Geometry: final body of the model. Coordinates: model frame, mm. Face numbers are marked on the shaded views. A direction names the side the tool comes from. Give positions to 0.01 mm unless a question says otherwise; leave off trailing zeros. Order: outer loops, then holes, each group sorted by start corner. A loop starts at its lowest first (then second) coordinate and runs counter-clockwise, first axis right, second up. Notation, with made-up numbers: (4.25, -16) - (42.25, -16) arc R11 ccw to (42.25, -1) - close; hole circle Ø6 at (33.25, 57). An arc over 180 degrees is marked (long way). One line per item, written item: value.
```python
from build123d import *

# Parameters (mm, degrees)
SKETCH1_R                       = 15.5
BASE_FLANGE1_DEPTH              = 2
EDGE_FLANGE1_STRIP_W            = 9.4732
EDGE_FLANGE1_STRIP_H            = 2
EDGE_FLANGE1_STRIP_CUT_DEPTH    = 40
EDGE_FLANGE1_RELIEF_W           = 10.4732
EDGE_FLANGE1_RELIEF_H           = 1
EDGE_FLANGE1_RELIEF_CUT_DEPTH   = 2
EDGE_FLANGE1_STRIP_2_W          = 9.4732
EDGE_FLANGE1_STRIP_2_H          = 2
EDGE_FLANGE1_STRIP_CUT_2_DEPTH  = 40
EDGE_FLANGE1_RELIEF_2_W         = 10.4732
EDGE_FLANGE1_RELIEF_2_H         = 1
EDGE_FLANGE1_RELIEF_CUT_2_DEPTH = 2
EDGE_FLANGE1_DEPTH              = 40
EDGE_FLANGE1_BEND_DEPTH         = 40
EDGE_FLANGE2_STRIP_W            = 9.4732
EDGE_FLANGE2_STRIP_H            = 2
EDGE_FLANGE2_STRIP_CUT_DEPTH    = 40
EDGE_FLANGE2_STRIP_2_W          = 9.4732
EDGE_FLANGE2_STRIP_2_H          = 2
EDGE_FLANGE2_STRIP_CUT_2_DEPTH  = 40
EDGE_FLANGE2_DEPTH              = 40
EDGE_FLANGE2_BEND_DEPTH         = 40
SKETCH17_R                      = 3
CUT_EXTRUDE1_DEPTH              = 10
FILLET1_R                       = 2


# Sheet-metal steps are written as plain solids
with BuildPart() as part:
    # Sketch1 → Base-Flange1 (new body)
    with BuildSketch(Plane.XY):
        with BuildLine():
            Line((-31, 20), (-11.034132012, 27.897095382))
            ThreePointArc((-11.034132012, 27.897095382), (0, 30), (11.034132012, 27.897095382))
            Line((11.034132012, 27.897095382), (31, 20))
            Line((31, 20), (31, -20))
            Line((31, -20), (11.034132012, -27.897095382))
            ThreePointArc((11.034132012, -27.897095382), (0, -30), (-11.034132012, -27.897095382))
            Line((-11.034132012, -27.897095382), (-31, -20))
            Line((-31, -20), (-31, 20))
        make_face()
        Circle(SKETCH1_R, mode=Mode.SUBTRACT)
    extrude(amount=-BASE_FLANGE1_DEPTH)

    # Edge-Flange1 strip (across the edge) → Edge-Flange1 strip cut (cut)
    with BuildSketch(Plane(origin=(-31, 20, 0), x_dir=(1, 0, 0), z_dir=(0, -1, 0))):
        with Locations((-4, -1)):
            Rectangle(EDGE_FLANGE1_STRIP_W, EDGE_FLANGE1_STRIP_H)
    extrude(amount=EDGE_FLANGE1_STRIP_CUT_DEPTH, mode=Mode.SUBTRACT)

    # Edge-Flange1 relief (on the sheet) → Edge-Flange1 relief cut (cut)
    with BuildSketch(Plane(origin=(-30.2634, 20, 0), x_dir=(1, 0, 0), z_dir=(0, 0, 1))):
        with Locations((-4.2366, 0.5)):
            Rectangle(EDGE_FLANGE1_RELIEF_W, EDGE_FLANGE1_RELIEF_H)
        with Locations((-4.2366, -40.5)):
            Rectangle(EDGE_FLANGE1_RELIEF_W, EDGE_FLANGE1_RELIEF_H)
    extrude(amount=-EDGE_FLANGE1_RELIEF_CUT_DEPTH, mode=Mode.SUBTRACT)

    # Edge-Flange1 strip 2 (across the edge) → Edge-Flange1 strip cut 2 (cut)
    with BuildSketch(Plane(origin=(31, -20, 0), x_dir=(-1, 0, 0), z_dir=(0, 1, 0))):
        with Locations((-4, -1)):
            Rectangle(EDGE_FLANGE1_STRIP_2_W, EDGE_FLANGE1_STRIP_2_H)
    extrude(amount=EDGE_FLANGE1_STRIP_CUT_2_DEPTH, mode=Mode.SUBTRACT)

    # Edge-Flange1 relief 2 (on the sheet) → Edge-Flange1 relief cut 2 (cut)
    with BuildSketch(Plane(origin=(30.2634, -20, 0), x_dir=(-1, 0, 0), z_dir=(0, 0, 1))):
        with Locations((-4.2366, 0.5)):
            Rectangle(EDGE_FLANGE1_RELIEF_2_W, EDGE_FLANGE1_RELIEF_2_H)
        with Locations((-4.2366, -40.5)):
            Rectangle(EDGE_FLANGE1_RELIEF_2_W, EDGE_FLANGE1_RELIEF_2_H)
    extrude(amount=-EDGE_FLANGE1_RELIEF_CUT_2_DEPTH, mode=Mode.SUBTRACT)

    # Edge-Flange1 section (across the edge) → Edge-Flange1 (add)
    with BuildSketch(Plane(origin=(-31, 20, 0), x_dir=(1, 0, 0), z_dir=(0, -1, 0))):
        with BuildLine():
            Line((-2, 0.7366), (-2, 28))
            Line((-2, 28), (0, 28))
            Line((0, 28), (0, 0.7366))
            ThreePointArc((0, 0.7366), (0.215745145, 0.215745145), (0.7366, 0))
            Line((0.7366, 0), (0.7366, -2))
            ThreePointArc((0.7366, -2), (-1.198468417, -1.198468417), (-2, 0.7366))
        make_face()
    extrude(amount=EDGE_FLANGE1_DEPTH)

    # Edge-Flange1 section 2 (across the edge) → Edge-Flange1 bend (add)
    with BuildSketch(Plane(origin=(31, -20, 0), x_dir=(-1, 0, 0), z_dir=(0, 1, 0))):
        with BuildLine():
            Line((-2, 0.7366), (-2, 28))
            Line((-2, 28), (0, 28))
            Line((0, 28), (0, 0.7366))
            ThreePointArc((0, 0.7366), (0.215745145, 0.215745145), (0.7366, 0))
            Line((0.7366, 0), (0.7366, -2))
            ThreePointArc((0.7366, -2), (-1.198468417, -1.198468417), (-2, 0.7366))
        make_face()
    extrude(amount=EDGE_FLANGE1_BEND_DEPTH)

    # Edge-Flange2 strip (across the edge) → Edge-Flange2 strip cut (cut)
    with BuildSketch(Plane(origin=(-33, -20, 28), x_dir=(0, 0, -1), z_dir=(0, 1, 0))):
        with Locations((-4, -1)):
            Rectangle(EDGE_FLANGE2_STRIP_W, EDGE_FLANGE2_STRIP_H)
    extrude(amount=EDGE_FLANGE2_STRIP_CUT_DEPTH, mode=Mode.SUBTRACT)

    # Edge-Flange2 strip 2 (across the edge) → Edge-Flange2 strip cut 2 (cut)
    with BuildSketch(Plane(origin=(33, 20, 28), x_dir=(0, 0, -1), z_dir=(0, -1, 0))):
        with Locations((-4, -1)):
            Rectangle(EDGE_FLANGE2_STRIP_2_W, EDGE_FLANGE2_STRIP_2_H)
    extrude(amount=EDGE_FLANGE2_STRIP_CUT_2_DEPTH, mode=Mode.SUBTRACT)

    # Edge-Flange2 section (across the edge) → Edge-Flange2 (add)
    with BuildSketch(Plane(origin=(-33, -20, 28), x_dir=(0, 0, -1), z_dir=(0, 1, 0))):
        with BuildLine():
            Line((-2, 0.7366), (-2, 32))
            Line((-2, 32), (0, 32))
            Line((0, 32), (0, 0.7366))
            ThreePointArc((0, 0.7366), (0.215745145, 0.215745145), (0.7366, 0))
            Line((0.7366, 0), (0.7366, -2))
            ThreePointArc((0.7366, -2), (-1.198468417, -1.198468417), (-2, 0.7366))
        make_face()
    extrude(amount=EDGE_FLANGE2_DEPTH)

    # Edge-Flange2 section 2 (across the edge) → Edge-Flange2 bend (add)
    with BuildSketch(Plane(origin=(33, 20, 28), x_dir=(0, 0, -1), z_dir=(0, -1, 0))):
        with BuildLine():
            Line((-2, 0.7366), (-2, 32))
            Line((-2, 32), (0, 32))
            Line((0, 32), (0, 0.7366))
            ThreePointArc((0, 0.7366), (0.215745145, 0.215745145), (0.7366, 0))
            Line((0.7366, 0), (0.7366, -2))
            ThreePointArc((0.7366, -2), (-1.198468417, -1.198468417), (-2, 0.7366))
        make_face()
    extrude(amount=EDGE_FLANGE2_BEND_DEPTH)

    # Sketch17 → Cut-Extrude1 (cut)
    with BuildSketch(Plane(origin=(0, 0, 28), x_dir=(-1, 0, 0), z_dir=(0, 0, -1))):
        with Locations((60, 0)):
            Circle(SKETCH17_R)
        with Locations((42, 0)):
            Circle(SKETCH17_R)
        with Locations((-60, 0)):
            Circle(SKETCH17_R)
        with Locations((-42, 0)):
            Circle(SKETCH17_R)
    extrude(amount=-CUT_EXTRUDE1_DEPTH, mode=Mode.SUBTRACT)

    # Fillet1
    fillet1_edges = [part.edges().sort_by_distance(p)[0] for p in [
        (-65, -20, 29),
        (-65, 20, 29),
        (65, 20, 29),
        (65, -20, 29),
    ]]
    fillet(fillet1_edges, radius=FILLET1_R)


solid = part.part
```
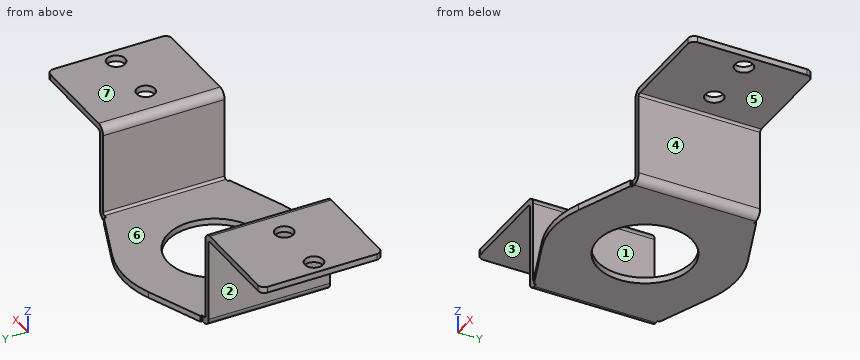
1) Section B-B, the plane z = 2. Return loops of the section in (x, y), then the cut area to 3 significant figures.
Answers below:
outline: (-33, -20) - (-31, -20) - (-31, 20) - (-33, 20) - close; (31, -20) - (33, -20) - (33, 20) - (31, 20) - close
area: 160 mm^2
2) Set-up query: the marked faces 5, 6 and 7. Return all of +Z, -Z, +X, -X, +Y, -Y with unobstructed straight access to the full face (end or side cutting, diameter ignored); none if empty.
Answers below:
face 5: -Z, +X, +Y, -Y
face 6: +Z, +Y, -Y
face 7: +Z, +X, -X, +Y, -Y
3) Material intervals for line 1 along X through (y, z) = (2.5, 1); line 2 along Y through (x, z) = (42, 29.5); line 3 along Z through (x, y) = (47.5, 6.5), sorted ascending.
Answers below:
line 1: -33 to -31, 31 to 33
line 2: -20 to -3, 3 to 20
line 3: 28 to 30
4) Mould query, pull axis X, two halves, no side actions, for the marked faces 1, 2, 3 and 4. Classes: released by +X, released by -X, zero draft, split by the parting line, or undercut.
Answers below:
face 1: undercut
face 2: released by -X
face 3: zero draft
face 4: released by +X
5) Section C-C, the plane y = -14. Return loops of the section in (x, z).
Answers below:
outline: (-65, 28) - (-33.74, 28) arc R0.74 cw to (-33, 27.26) - (-33, 0.74) arc R2.74 ccw to (-30.26, -2) - (-6.65, -2) - (-6.65, 0) - (-30.26, 0) arc R0.74 cw to (-31, 0.74) - (-31, 27.26) arc R2.74 ccw to (-33.74, 30) - (-65, 30) - close; (6.65, -2) - (30.26, -2) arc R2.74 ccw to (33, 0.74) - (33, 27.26) arc R0.74 cw to (33.74, 28) - (65, 28) - (65, 30) - (33.74, 30) arc R2.74 ccw to (31, 27.26) - (31, 0.74) arc R0.74 cw to (30.26, 0) - (6.65, 0) - close
6) First-contact query: pin 1 (10 mm diameter, centred on x = 35.5, y = 14.5, fed in from -Z); pin 2 (7 mm diameter, centred on x = -42, y = 0, fed in from -Z); pin 3 (0.8 mm diameter, centred on y = -20, z = -0.5, fed in from -X); pin 4 (9.5 mm diameter, centred on x = -38.5, z = 15.5, fed in from +Y). Flat tips, straight axial feed; report the tip coordinate or a pass-through.
Answers below:
pin 1: z = -1.99
pin 2: z = 28
pin 3: x = -32.87
pin 4: through
7) Section A-A, the plane x = -60. Return loops of the section in (y, z).
Answers below:
outline: (-20, 28) - (-3, 28) - (-3, 30) - (-20, 30) - close; (3, 28) - (20, 28) - (20, 30) - (3, 30) - close
8) Section D-D, the plane y = -5.5. Return loops of the section in (x, z).
Answers below:
outline: (-65, 28) - (-33.74, 28) arc R0.74 cw to (-33, 27.26) - (-33, 0.74) arc R2.74 ccw to (-30.26, -2) - (-14.49, -2) - (-14.49, 0) - (-30.26, 0) arc R0.74 cw to (-31, 0.74) - (-31, 27.26) arc R2.74 ccw to (-33.74, 30) - (-65, 30) - close; (14.49, -2) - (30.26, -2) arc R2.74 ccw to (33, 0.74) - (33, 27.26) arc R0.74 cw to (33.74, 28) - (65, 28) - (65, 30) - (33.74, 30) arc R2.74 ccw to (31, 27.26) - (31, 0.74) arc R0.74 cw to (30.26, 0) - (14.49, 0) - close
